The drawing under review shows one solid part. Ordinate dimensions are in mm from its lowest x, y, z. A direction names the side the tool comes from. Coordinates: 2 decimals unless noted, no trailing zeros. Write each loop counter-clockwise with the first axis right and the second up, starting at its lowest first coordinate (ties: lowest second). Pieces come first, ordered by that corner, then holes. Notation, with made-up numbers: (47.5, 46) -> (65.5, 46) arc R19 cw to (65.5, 65) -> close; hole circle Ø10 at (31.5, -26). An arc over 180 degrees is marked (long way). Put each result on its own line as item: value. Start each with the question number.
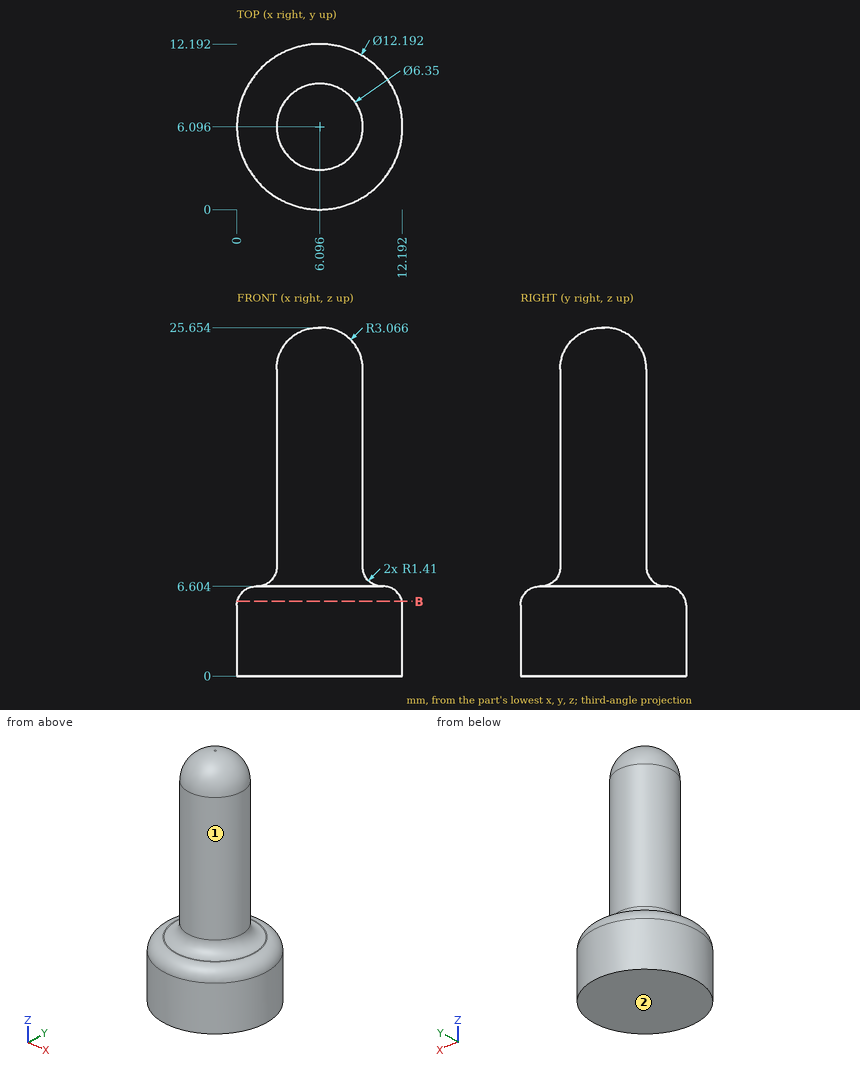
1. Tool access review of the marked faces 1 and 2: name each direction out of +Z, -Z, +X, -X, +Y, -Y from which nothing blocks a thin tool from reaching the whole face with its end or side.
2. Consider section B-B on z = 5.5. State the section outline as (x, y) points (1 decimal), then the cut area to 3 significant figures.
3. Wall thickness on line 1 (Z direction, x = 1.75, y = 2.25) (1 decimal); line 2 (Z direction, x = 4.5, y = 6.5); line 3 (Y direction, x = 1.5, z = 4.25): over which ranges is each line inside the solid? List them lowest first. Write a range as from..to.
4. Insertion check: P1, Ø6, axis at x = 7.5, z = 16.5, coming from the -Y side; P2, Ø1.5, axis at y = 7.5, z = 14, coming from the -X side; P3, Ø4, axis at x = 7.5, z = 7.5, coming from the +Y side. Each pin has a flat end and moves straight along its axis. Give the tip position at first contact, or say it passes through.
Output values:
1. face 1: +Z
1. face 2: -Z, +X, -X, +Y, -Y
2. outline: circle Ø12.1 at (6.1, 6.1)
2. area: 115 mm^2
3. line 1: z = 0..6.1
3. line 2: z = 0..25.24
3. line 3: y = 2.09..10.1
4. P1: stops at y = 2.92
4. P2: stops at x = 2.99
4. P3: stops at y = 12.08
